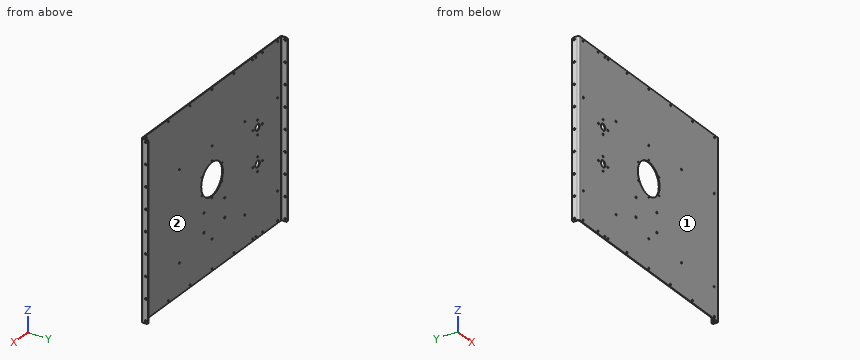
from build123d import *

# Parameters (mm, degrees)
BASE_FLANGE1_DEPTH       = 325
F_7_0_7_DIAMETER_HOLE1_D = 7
M5_CLEARANCE_HOLE1_D     = 5.8
SKETCH6_R                = 60
CUT_EXTRUDE1_DEPTH       = 3
M4_CLEARANCE_HOLE1_D     = 4.5
M6_CLEARANCE_HOLE1_D     = 6.6
M5_CLEARANCE_HOLE4_D     = 5.8
SKETCH13_R               = 12
CUT_EXTRUDE2_DEPTH       = 3
M5_CLEARANCE_HOLE2_D     = 5.8
M5_CLEARANCE_HOLE3_D     = 5.8
FILLET1_R                = 5


# Sheet-metal steps are written as plain solids
with BuildPart() as part:
    # Base-Flange1: sheet metal written as solids
    # Sketch1 → Base-Flange1 (new, symmetric)
    with BuildSketch(Plane.XY):
        with BuildLine():
            Line((-387.5, 25), (-387.5, 6))
            ThreePointArc((-387.5, 6), (-385.742640687, 1.757359313), (-381.5, 0))
            Line((-381.5, 0), (381.5, 0))
            ThreePointArc((381.5, 0), (385.742640687, 1.757359313), (387.5, 6))
            Line((387.5, 6), (387.5, 25))
            Line((387.5, 25), (384.5, 25))
            Line((384.5, 25), (384.5, 6))
            ThreePointArc((384.5, 6), (383.621320344, 3.878679656), (381.5, 3))
            Line((381.5, 3), (-381.5, 3))
            ThreePointArc((-381.5, 3), (-383.621320344, 3.878679656), (-384.5, 6))
            Line((-384.5, 6), (-384.5, 25))
            Line((-384.5, 25), (-387.5, 25))
        make_face()
    extrude(amount=BASE_FLANGE1_DEPTH, both=True)

    # Ø7.0 (7) Diameter Hole1 (through all)
    with Locations(Plane(origin=(387.5, 0, 0), x_dir=(0, 0, -1), z_dir=(1, 0, 0))):
        with Locations((-316.5, 16.5), (-237.375, 16.5), (-158.25, 16.5), (-79.125, 16.5), (0, 16.5), (79.125, 16.5), (158.25, 16.5), (237.375, 16.5), (316.5, 16.5)):
            Hole(F_7_0_7_DIAMETER_HOLE1_D / 2)

    # M5 Clearance Hole1 (through all)
    with Locations(Plane(origin=(0, 0, 0), x_dir=(-1, 0, 0), z_dir=(0, -1, 0))):
        with Locations((-363.5, 316.5), (-242.333333333, 316.5), (-121.166666667, 316.5), (0, 316.5), (121.166666667, 316.5), (242.333333333, 316.5), (363.5, 316.5)):
            m5_clearance_hole1 = Hole(M5_CLEARANCE_HOLE1_D / 2)

    # Mirror1: M5 Clearance Hole1 across plane
    add(m5_clearance_hole1.mirror(Plane.XY), mode=Mode.SUBTRACT)

    # Sketch6 → Cut-Extrude1 (cut)
    with BuildSketch(Plane(origin=(0, 3, 0), x_dir=(1, 0, 0), z_dir=(0, 1, 0))):
        with Locations(Location((0, 0, 0), (0, 0, 270))):
            Circle(SKETCH6_R)
    extrude(amount=-CUT_EXTRUDE1_DEPTH, mode=Mode.SUBTRACT)

    # M4 Clearance Hole1 (through all)
    with Locations(Plane(origin=(0, 3, 0), x_dir=(1, 0, 0), z_dir=(0, 1, 0))):
        with Locations((0, -65.5), (-56.724663948, -32.75), (-56.724663948, 32.75), (0, 65.5), (56.724663948, 32.75), (56.724663948, -32.75)):
            Hole(M4_CLEARANCE_HOLE1_D / 2)

    # M6 Clearance Hole1 (through all)
    with Locations(Plane(origin=(0, 3, 0), x_dir=(1, 0, 0), z_dir=(0, 1, 0))):
        with Locations((-70.35, 168.5), (44.65, 168.5), (-70.35, 98.5), (44.65, 98.5)):
            Hole(M6_CLEARANCE_HOLE1_D / 2)

    # M5 Clearance Hole4 (through all)
    with Locations(Plane(origin=(0, 3, 0), x_dir=(1, 0, 0), z_dir=(0, 1, 0))):
        with Locations((-362.5, 211.5), (-181.25, 211.5), (0, 211.5), (181.25, 211.5), (362.5, 211.5), (181.25, -118), (362.5, -118), (0, -118), (-181.25, -118), (-362.5, -118)):
            Hole(M5_CLEARANCE_HOLE4_D / 2)

    # Sketch13 → Cut-Extrude2 (cut)
    with BuildSketch(Plane(origin=(0, 3, 0), x_dir=(1, 0, 0), z_dir=(0, 1, 0))):
        with Locations(Location((-252.5, 65, 0), (0, 0, 270))):
            Circle(SKETCH13_R)
        with Locations(Location((-252.5, -65, 0), (0, 0, 270))):
            Circle(SKETCH13_R)
    extrude(amount=-CUT_EXTRUDE2_DEPTH, mode=Mode.SUBTRACT)

    # M5 Clearance Hole2 (through all)
    with Locations(Plane(origin=(0, 3, 0), x_dir=(1, 0, 0), z_dir=(0, 1, 0))):
        with Locations((-278.5, 65), (-252.5, 91), (-252.5, 39), (-226.5, 65), (-278.5, -65), (-226.5, -65), (-252.5, -91), (-252.5, -39)):
            Hole(M5_CLEARANCE_HOLE2_D / 2)

    # M5 Clearance Hole3 (through all)
    with Locations(Plane(origin=(0, 3, 0), x_dir=(1, 0, 0), z_dir=(0, 1, 0))):
        with Locations((-280, 316.5), (-225, 316.5), (-280, -316.5), (-225, -316.5)):
            Hole(M5_CLEARANCE_HOLE3_D / 2)

    # Fillet1
    fillet1_edges = [part.edges().sort_by_distance(p)[0] for p in [
        (-386, 25, -325),
        (386, 25, -325),
        (-386, 25, 325),
        (386, 25, 325),
    ]]
    fillet(fillet1_edges, radius=FILLET1_R)


solid = part.part
Geometry: final body of the model. Coordinates: model frame, mm. Face numbers are marked on the shaded views. Give positions to 0.01 mm unless a question says otherwise; leave off trailing zeros. Loops run counter-clockwise (first coordinate to the right, second up) from the corner with the lowest first, then second, coordinate; pieces in that order, holes last. Notation, with made-up numbers: (63.25, 78.25) - (119.25, 78.25) arc R13 cw to (119.25, 85.25) - close; hole circle Ø9 at (82, 49). An arc over 180 degrees is marked (long way). One line per question, with ' | ' between items. Start each with the question number.
(1) Pull-direction query (X, two-part tool) for the marked faces 1 and 2; classes: released by +X, released by -X, zero draft, split by the parting line, or undercut.
(2) Contact query for a flat-ended pin moving along its axis: pin 1 (7.5 mm diameter, centred on x = -70.35, z = -168.5, fed in from +Y). Output: stop coordinate, or through.
(3) Section query A-A on x = -339. Return loops of the section in (y, z).
(4) Ray query, line 1 (Z direction, x = 362.5, y = 1.3); line 2 (X direction, y = 16.75, z = -215); line 3 (Z direction, x = -226.5, y = 1.4). Return the intervals inside material, ascending. Write a range as from..to.
The answers:
1) face 1: zero draft | face 2: undercut
2) pin 1: y = 3
3) outline: (0, -325) - (3, -325) - (3, 325) - (0, 325) - close
4) line 1: -325..-319.22, -313.78..-214.4, -208.6..115.1, 120.9..313.78, 319.22..325 | line 2: -387.5..-384.5, 384.5..387.5 | line 3: -325..-318.98, -314.02..-67.9, -62.1..62.1, 67.9..314.02, 318.98..325
